from build123d import *

# Parameters (mm, degrees)
F0_R      = 16.25
F1_DEPTH  = 15.875
F2_W      = 139.2096877098
F2_H      = 115.5483946204
F2_W_2    = 113
F2_H_2    = 80
F3_DEPTH  = 5.875
F4_W      = 107
F4_H      = 80
F5_DEPTH  = 14
F6_W      = 120.5911301091
F6_H      = 13.1527084535
F6_W_2    = 121.3300417974
F6_H_2    = 15.8128053223
F7_DEPTH  = 5.875
F8_R      = 1.5
F8_W      = 89
F8_H      = 3
F9_DEPTH  = 100
F10_W     = 42.4407012761
F10_H     = 10
F11_DEPTH = 1.5
F12_W     = 42.5221920013
F12_H     = 10
F13_DEPTH = 1.5
F14_R     = 2.5
F15_DEPTH = 95.5
F16_R     = 2.25
F17_DEPTH = 200
F18_R     = 5
F19_R     = 1.5
F20_DEPTH = 106.2
F21_R     = 1.5
F22_DEPTH = 121.8


with BuildPart() as f1:
    # F0 (on Front) → F1 (new body)
    with BuildSketch(Plane.XZ):
        Polygon((-50.5, 47.5), (-62.5, 47.5), (-62.5, -47.5), (-50.5, -47.5), (-50.5, -41.5), (50.5, -41.5), (50.5, -47.5), (62.5, -47.5), (62.5, 47.5), (50.5, 47.5), (50.5, 41.5), (-50.5, 41.5), align=None)
        Circle(F0_R, mode=Mode.SUBTRACT)
    extrude(amount=F1_DEPTH)

    # F2 (on face) → F3 (cut)
    with BuildSketch(Plane.XZ.offset(15.875)):
        Rectangle(F2_W, F2_H)
        Rectangle(F2_W_2, F2_H_2, mode=Mode.SUBTRACT)
    extrude(amount=-F3_DEPTH, mode=Mode.SUBTRACT)

    # F4 (on face) → F5 (cut)
    with BuildSketch(Plane.XZ.offset(15.875)):
        Rectangle(F4_W, F4_H)
    extrude(amount=-F5_DEPTH, mode=Mode.SUBTRACT)

    # F6 (on face) → F7 (cut)
    with BuildSketch(Plane.XZ.offset(15.875)):
        with Locations((0.0607829645, 36.5763542267)):
            Rectangle(F6_W, F6_H)
        with Locations((1.0213727103, -37.9064026611)):
            Rectangle(F6_W_2, F6_H_2)
    extrude(amount=-F7_DEPTH, mode=Mode.SUBTRACT)

    # F8 (on face) → F9 (cut)
    with BuildSketch(Plane.XY.offset(41.5)):
        with Locations((46, -5.5)):
            Circle(F8_R)
        with Locations((-3, -5.5)):
            Rectangle(F8_W, F8_H)
    extrude(amount=-F9_DEPTH, mode=Mode.SUBTRACT)

    # F10 (on face) → F11 (join)
    with BuildSketch(Plane.XY.offset(41.5)):
        with Locations((21.220350638, -5)):
            Rectangle(F10_W, F10_H)
    extrude(amount=-F11_DEPTH)

    # F12 (on face) → F13 (join)
    with BuildSketch(Plane(origin=(0, 0, -41.5), x_dir=(1, 0, 0), z_dir=(0, 0, -1))):
        with Locations((21.2610960007, 5)):
            Rectangle(F12_W, F12_H)
    extrude(amount=-F13_DEPTH)

    # F14 (on face) → F15 (cut)
    with BuildSketch(Plane(origin=(0, 0, -41.5), x_dir=(1, 0, 0), z_dir=(0, 0, -1))):
        with Locations((39.25, 10)):
            Circle(F14_R)
    extrude(amount=-F15_DEPTH, mode=Mode.SUBTRACT)

    # F16 (on face) → F17 (cut)
    with BuildSketch(Plane.XY.offset(41.5)):
        with Locations((46, -5.5)):
            Circle(F16_R)
    extrude(amount=-F17_DEPTH, mode=Mode.SUBTRACT)

    # F18
    f18_edges = [f1.edges().sort_by_distance(p)[0] for p in [
        (41.75, -10, -40.75),
        (41.75, -10, 40.75),
    ]]
    fillet(f18_edges, radius=F18_R)

    # F19 (on face) → F20 (cut)
    with BuildSketch(Plane.XY.offset(47.5)):
        with Locations((-56.5, -5)):
            Circle(F19_R)
    extrude(amount=-F20_DEPTH, mode=Mode.SUBTRACT)

    # F21 (on face) → F22 (cut)
    with BuildSketch(Plane.XY.offset(47.5)):
        with Locations((56.5, -5)):
            Circle(F21_R)
    extrude(amount=-F22_DEPTH, mode=Mode.SUBTRACT)


solid = f1.part
The model under review builds one solid part; all positions refer to its coordinate system, in mm. A direction names the side the tool comes from. Round coordinates to 2 decimals unless told otherwise and drop trailing zeros. Write each loop counter-clockwise with the first axis right and the second up, starting at its lowest first coordinate (ties: lowest second). Pieces come first, ordered by that corner, then holes. Notation, with made-up numbers: (-37.75, 87.5) -> (-31.75, 87.5) arc R21 ccw to (-31.75, 97.5) -> close; hole circle Ø9 at (47, -30). An arc over 180 degrees is marked (long way). Answer as a JSON object with one key per item and string values.
1. The part is to be moulded in two halves that separate along Y. For faces 5 (the face through (43.752, -5.401, -40.74)), 6 (the face through (55, -13, -30)), 7 (the face through (38.32, -7.68, 40.74)), say which applies: pulls with the +Y half, pulls with the -Y half, needs draft (parallel to the pull), parting line crosses it, or undercut.
Results found:
{"face 5": "undercut", "face 6": "needs draft", "face 7": "pulls with the -Y half"}
2. Machinability: for faces 1 (the face through (-55, -13, 30)), 2 (the face through (56.5, -13, 0)), 3 (the face through (-1, -8, 40)), 4 (the face through (-56.5, -13, 0)), which of the approach directions +Z, -Z, +X, -X, +Y, -Y give a long, thin tool a straight path to every point of the face, cutting with its end or side? Answer none if there is none.
Results found:
{"face 1": "+Z, +X, -X, -Y", "face 2": "+Z, -Z, +X, -Y", "face 3": "-Y", "face 4": "+Z, -Z, -X, -Y"}
3. We need section C-C on x = 23. State the section outline as (y, z) points (3 decimals).
Results found:
{"outline": "(-10, -41.5) -> (0, -41.5) -> (0, 41.5) -> (-10, 41.5) -> (-10, 40) -> (-1.875, 40) -> (-1.875, -40) -> (-10, -40) -> close"}
4. To check wall thickness, follow line 1 along X through (y, z) = (-5.25, -17); line 2 along Z through (x, y) = (-32.5, -2); line 3 along X through (y, z) = (-9.75, 33). State the ranges of each line that lie inside material, in increasing order.
Results found:
{"line 1": "x = -62.5 to -57.98, -55.02 to -53.5, 53.5 to 55.02, 57.98 to 62.5", "line 2": "z = -41.5 to -40, 40 to 41.5", "line 3": "x = -62.5 to -53.5, 53.5 to 62.5"}
5. Clearance check with flat-ended pins moving along their axes: pin 1 (5 mm diameter, centred on x = -37, z = 10, fed in from -Y) (3 decimals); pin 2 (3 mm diameter, centred on x = -16, y = -6.5, fed in from -Z); pin 3 (2 mm diameter, centred on x = 29, y = -3.5, fed in from +Z). State where each tip first meets the part, or that it passes through.
Results found:
{"pin 1": "stops at y = -1.875", "pin 2": "stops at z = -41.5", "pin 3": "stops at z = 41.5"}
6. We need section A-A on x = -37.5. State the section outline as (y, z) points (3 decimals), and give its area (3 significant figures).
Results found:
{"outline": "(-10, -41.5) -> (-7, -41.5) -> (-7, -40) -> (-10, -40) -> close; (-10, 40) -> (-7, 40) -> (-7, 41.5) -> (-10, 41.5) -> close; (-4, -41.5) -> (0, -41.5) -> (0, 41.5) -> (-4, 41.5) -> (-4, 40) -> (-1.875, 40) -> (-1.875, -40) -> (-4, -40) -> close", "area": "171 mm^2"}
7. We need section B-B on z = 25.5. State the section outline as (x, y) points (3 decimals), and give its area (3 significant figures).
Results found:
{"outline": "(-62.5, -10) -> (-56.5, -10) -> (-56.5, -15.875) -> (-53.5, -15.875) -> (-53.5, -1.875) -> (53.5, -1.875) -> (53.5, -15.875) -> (56.5, -15.875) -> (56.5, -10) -> (62.5, -10) -> (62.5, 0) -> (-62.5, 0) -> close; hole circle Ø3 at (-56.5, -5); hole circle Ø3 at (56.5, -5)", "area": "402 mm^2"}
